The listing builds one solid part. Answer for the finished solid, in the listing's coordinates (mm). Face numbers are marked on the shaded views. A direction names the side the tool comes from. Give positions to 0.01 mm unless a question says otherwise; leave off trailing zeros. Write each loop counter-clockwise with the first axis right and the second up, starting at its lowest first coordinate (ties: lowest second). Pieces come first, ordered by that corner, then holes.
Autodesk Inventor part; units mm, degrees
ref_plane "YZ Plane" through (0, 0, 0) normal (1, 0, 0) x (0, 1, 0)
ref_plane "XZ Plane" through (0, 0, 0) normal (0, 1, 0) x (-1, 0, 0)
ref_plane "XY Plane" through (0, 0, 0) normal (0, 0, 1) x (1, 0, 0)
sketch "Sketch1" plane through (0, 0, 0) normal (0, 1, 0) x (-1, 0, 0)
  line L0 (0, 0) -> (25.4, 0)
  line L1 (25.4, 0) -> (25.4, 127)
  line L2 (25.4, 127) -> (0, 127)
  line L3 (0, 127) -> (0, 0)
  dimension "d0" = 25.4
  dimension "d1" = 127
extrude "Plate1" add sketch "Sketch1" along normal blind 3.175
sketch "Sketch2" plane through (-22.225, 0, 127) normal (-1, 0, 0) x (0, -1, 0)
  line L0 (0, -127) -> (0, 0)
  line L1 (0, 0) -> (-25.4, 0)
  line L2 (-25.4, 0) -> (-25.4, -127)
  line L3 (-25.4, -127) -> (0, -127)
edge flange "Flange1" height 25.4 angle 90 thickness 3.175 bend radius 4.7625 thickness toward (-1, 0, 0) relief tear relief width 3.175 relief depth 1.5875 edges at (-25.4, 3.175, 63.5) wall of the first edge with corners at (-22.225, 0, 0) (-22.225, 0, 127) (-22.225, 25.4, 127) (-22.225, 25.4, 0)
bend "Bend1"
corner "Corner1"
sketch "Sketch3" plane through (0, 3.175, 0) normal (0, 1, 0) x (1, 0, 0)
  line L0 (-17.4625, 0) -> (0, 0) construction
  line L1 (-8.7313, 0) -> (-8.7312, -127) construction
  line L2 (0, -127) -> (-17.4625, -127) construction
  point P0 (-8.7312, -12.7)
  point P1 (-8.7312, -114.3)
  dimension "d13" = 12.7
  dimension "d14" = 12.7
hole "Hole1" at (-8.7312, 3.175, 12.7) at (-8.7312, 3.175, 114.3) direction (0, -1, 0) diameter 4.0894 end through all
equation "\"d20\" = Thickness"
equation "\"d2\" = Thickness"
equation "\"d3\" = BendReliefWidth"
equation "\"d4\" = BendReliefDepth"
equation "\"d5\" = MinimumRemnant"
equation "\"d6\" = TransitionRadius"
equation "\"d9\" = BendRadius"
equation "\"d10\" = CornerReliefSize"
equation "\"d11\" = GapSize"
equation "\"d12\" = JacobiRadiusSize"
equation "\"BendRadius\" = 1.5 * Thickness"
equation "\"BendReliefWidth\" = Thickness"
equation "\"BendReliefDepth\" = 0.5 * Thickness"
equation "\"CornerReliefSize\" = 4 * Thickness"
equation "\"MinimumRemnant\" = 2 * Thickness"
equation "\"TransitionRadius\" = BendRadius"
equation "\"JacobiRadiusSize\" = BendRadius"
equation "\"GapSize\" = Thickness"
properties part number "200512" material "Aluminum 5052 H32"
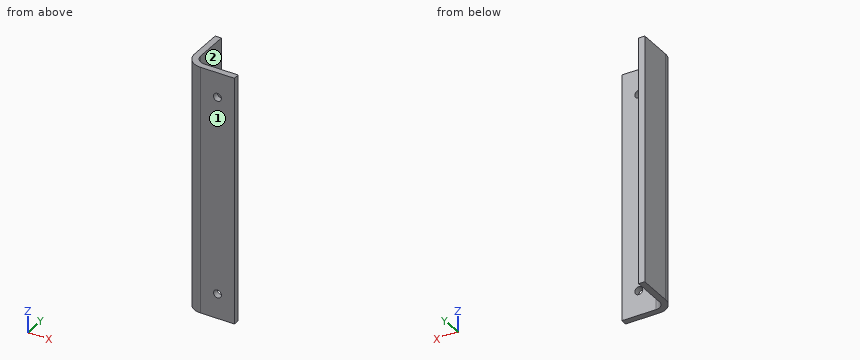
Item 1: A cutting plane is placed at B-B, the plane y = 17.5. Give the vertices of the cut face in (x, z) (3 decimals).
Conclusion:
outline: (-25.4, 0) - (-22.225, 0) - (-22.225, 127) - (-25.4, 127) - close
Item 2: Consider probe 1 along Y at (x, z) = (-5.25, 83.5) (3 decimals); probe 2 along X at (y, z) = (16.75, 71) (3 decimals); probe 3 along X at (y, z) = (0.8, 12.7). Determine where each line is inside the solid, lowest interval first.
Conclusion:
probe 1: y = 0 to 3.175
probe 2: x = -25.4 to -22.225
probe 3: x = -20.94 to -10.78, -6.69 to 0
Item 3: A cutting plane is placed at D-D, the plane x = -5.5. Give the vertices of the cut face in (y, z) (3 decimals).
Conclusion:
outline: (0, 0) - (3.175, 0) - (3.175, 127) - (0, 127) - close
Item 4: A cutting plane is placed at A-A, the plane z = 114.3. Give the vertices of the cut face in (x, y) (1 decimal).
Conclusion:
outline: (-25.4, 7.9) arc R7.9 ccw to (-17.5, 0) - (-10.8, 0) - (-10.8, 3.2) - (-17.5, 3.2) arc R4.8 cw to (-22.2, 7.9) - (-22.2, 25.4) - (-25.4, 25.4) - close; (-6.7, 0) - (0, 0) - (0, 3.2) - (-6.7, 3.2) - close
Item 5: A cutting plane is placed at C-C, the plane z = 39. Give the vertices of the cut face in (x, y) (1 decimal).
Conclusion:
outline: (-25.4, 7.9) arc R7.9 ccw to (-17.5, 0) - (0, 0) - (0, 3.2) - (-17.5, 3.2) arc R4.8 cw to (-22.2, 7.9) - (-22.2, 25.4) - (-25.4, 25.4) - close
Item 6: Each of these flat-tipped pins is pushed along its axis until it touches: P1, Ø4, axis at x = -9.5, z = 109, coming from the +Y side (3 decimals); P2, Ø8, axis at y = 15.5, z = 35.5, coming from the +X side (3 decimals); P3, Ø3.5, axis at x = -8.73, z = 114.3, coming from the +Y side; P4, Ø1, axis at x = -23, z = 35.5, coming from the -Y side. Where does it stop, or does it pass through?
Conclusion:
P1: stops at y = 3.175
P2: stops at x = -22.225
P3: passes through
P4: stops at y = 1.8
Item 7: Which of the six approach directions +Z, -Z, +X, -X, +Y, -Y give full straight-line access (tool end or side, diameter ignored) to the marked faces 1 and 2?
Conclusion:
face 1: +Z, -Z, +X, -X, -Y
face 2: +Z, -Z, +X, +Y
